Input: part model. Units: mm. Frame: model coordinates. Face numbers are marked on the shaded views. A direction names the side the tool comes from. Coordinates: 2 decimals unless noted, no trailing zeros. Order: outer loops, then holes, each group sorted by start corner. A loop starts at its lowest first (then second) coordinate and runs counter-clockwise, first axis right, second up. Notation, with made-up numbers: (77, 84.25) -> (99, 84.25) arc R33 ccw to (99, 113.25) -> close; hole circle Ø2 at (-28.75, 30). An arc over 180 degrees is marked (long way). Use one line per item in the form item = value. Start each with the question number.
1) Draft query along Z for the marked faces 5, 6, 7 and 8. Return one class per face: pulls with the +Z half, pulls with the -Z half, needs draft (parallel to the pull), parting line crosses it, or undercut.
2) Access query for the marked faces 1, 2, 3 and 4. Directions: +Z, -Z, +X, -X, +Y, -Y. A direction counts if a zero-diameter tool reaches every point of the face in a straight line with its end or side. Return the directions, or none.
3) Section query C-C on z = 25.5. Output: boundary loops of the cut face in (x, y) (3 decimals), then the cut area to 3 significant figures.
4) Pin query (flat end, axial travel): pin 1 (12 mm diameter, centred on y = 9.5, z = 20, fed in from -X); pin 2 (12 mm diameter, centred on y = 15, z = -1.5, fed in from -X); pin 3 (4 mm diameter, centred on x = 7.5, z = 14.47, fed in from -Y); pin 4 (4 mm diameter, centred on y = -6.5, z = 3.5, fed in from +X). Return the tip coordinate at first contact, or that it passes through.
5) Section query A-A on y = 5. Output: boundary loops of the cut face in (x, z), then the cut area to 4 significant figures.
6) Section query B-B on z = 4. Output: boundary loops of the cut face in (x, y) (3 decimals).
7) Ray query, line 1 along X through (y, z) = (15.5, -9); line 2 along Y through (x, z) = (-6.5, 26.5) (3 decimals); line 3 along X through (y, z) = (-4, -3.5). Return the intervals inside material, ascending.
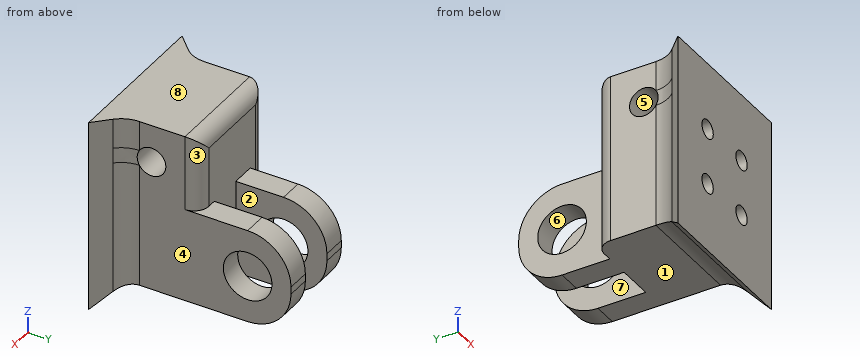
from build123d import *

# Parameters (mm, degrees)
SKETCH1_W                       = 28.58
SKETCH1_H                       = 50
BOSS_EXTRUDE1_DEPTH             = 12.5
SKETCH2_W                       = 9.53
SKETCH2_H                       = 24.225
SKETCH2_W_2                     = 6.35
CUT_EXTRUDE1_DEPTH              = 39.134028111
FILLET1_R                       = 11.53
SKETCH3_R                       = 6.477
CUT_EXTRUDE2_DEPTH              = 40.975822693
BOSS_EXTRUDE2_DEPTH             = 28.58
SKETCH5_W                       = 28.58
SKETCH5_H                       = 25.775
BOSS_EXTRUDE3_DEPTH             = 20
CUT_EXTRUDE3_DEPTH              = 50.98066026
CUT_EXTRUDE3_DEPTH_BACK         = 50.98066026
SKETCH6_R                       = 3.81
BOSS_EXTRUDE4_REACH             = 55.425
BOSS_EXTRUDE4_DIRECTION_2_REACH = 55.425
F_5_0MM_DOWEL_HOLE1_D           = 5
F_5_0MM_DOWEL_HOLE1_DEPTH       = 10
F_5_0MM_DOWEL_HOLE1_TIP         = 1.502151548
FILLET2_R                       = 8
FILLET4_R                       = 4


with BuildPart() as part:
    # Sketch1 → Boss-Extrude1 (new, symmetric)
    with BuildSketch(Plane.XY):
        Rectangle(SKETCH1_W, SKETCH1_H)
    extrude(amount=BOSS_EXTRUDE1_DEPTH, both=True)

    # Sketch2 → Cut-Extrude1 (cut, through all)
    with BuildSketch(Plane(origin=(0, 0, 12.5), x_dir=(-1, 0, 0), z_dir=(0, 0, 1))):
        with Locations((-3.175, -12.8875)):
            Rectangle(SKETCH2_W, SKETCH2_H)
        with Locations((11.115, -12.8875)):
            Rectangle(SKETCH2_W_2, SKETCH2_H)
    extrude(amount=-CUT_EXTRUDE1_DEPTH, mode=Mode.SUBTRACT)

    # Fillet1
    fillet1_edges = [part.edges().sort_by_distance(p)[0] for p in [
        (-4.765, 25, -12.5),
        (-4.765, 25, 12.5),
        (11.115, 25, -12.5),
        (11.115, 25, 12.5),
    ]]
    fillet(fillet1_edges, radius=FILLET1_R)

    # Sketch3 → Cut-Extrude2 (cut, through all)
    with BuildSketch(Plane(origin=(14.29, 0, 0), x_dir=(0, 0, -1), z_dir=(1, 0, 0))):
        with Locations(Location((0, 13.47, 0), (0, 0, 270))):
            Circle(SKETCH3_R)
    extrude(amount=-CUT_EXTRUDE2_DEPTH, mode=Mode.SUBTRACT)

    # Sketch4 → Boss-Extrude2 (add)
    with BuildSketch(Plane(origin=(14.29, 0, 0), x_dir=(0, 0, -1), z_dir=(1, 0, 0))):
        Polygon((18.85, -25), (12.5, -18.65), (12.5, -25), align=None)
    extrude(amount=-BOSS_EXTRUDE2_DEPTH)

    # Sketch5 → Boss-Extrude3 (add)
    with BuildSketch(Plane.XY.offset(12.5)):
        with Locations((0, -12.1125)):
            Rectangle(SKETCH5_W, SKETCH5_H)
    extrude(amount=BOSS_EXTRUDE3_DEPTH)

    # Sketch6 → Cut-Extrude3 (cut, two sides: drawn at the far end of the back side and taken through both)
    with BuildSketch(Plane(origin=(14.29, 0, 0), x_dir=(0, 0, -1), z_dir=(1, 0, 0)).offset(-CUT_EXTRUDE3_DEPTH_BACK)):
        with Locations((-22.5, -12.1125)):
            Circle(SKETCH6_R)
    extrude(amount=CUT_EXTRUDE3_DEPTH + CUT_EXTRUDE3_DEPTH_BACK, mode=Mode.SUBTRACT)

    # Boss-Extrude4: up to this face of the body (flat: up to its plane)
    boss_extrude4_end = Plane(part.part.faces().sort_by_distance((0, -12.1125, 32.5))[0])
    # Sketch7 → Boss-Extrude4 (add, up to the picked face)
    with BuildSketch(Plane(origin=(0, 0, -12.5), x_dir=(-1, 0, 0), z_dir=(0, 0, -1)), mode=Mode.PRIVATE) as boss_extrude4_sk1:
        Polygon((-14.29, -25), (-20.64, -25), (-14.29, -18.65), align=None)
    boss_extrude4_tool1 = split(extrude(boss_extrude4_sk1.sketch, amount=-BOSS_EXTRUDE4_REACH, mode=Mode.PRIVATE), bisect_by=boss_extrude4_end, keep=Keep.BOTH, mode=Mode.PRIVATE)
    boss_extrude4 = boss_extrude4_tool1.solids().sort_by(Axis((16.406667, -22.883333, -12.5), (0, 0, 1)))[0]
    add(boss_extrude4)

    # Boss-Extrude4 direction 2: up to this face of the body (flat: up to its plane)
    boss_extrude4_direction_2_end = Plane(part.part.faces().sort_by_distance((0, -21.825, -15.675))[0])
    # Sketch7 → Boss-Extrude4 direction 2 (add, up to the picked face)
    with BuildSketch(Plane(origin=(0, 0, -12.5), x_dir=(-1, 0, 0), z_dir=(0, 0, -1)), mode=Mode.PRIVATE) as boss_extrude4_direction_2_sk1:
        Polygon((-14.29, -25), (-20.64, -25), (-14.29, -18.65), align=None)
    boss_extrude4_direction_2_tool1 = split(extrude(boss_extrude4_direction_2_sk1.sketch, amount=BOSS_EXTRUDE4_DIRECTION_2_REACH, mode=Mode.PRIVATE), bisect_by=boss_extrude4_direction_2_end, keep=Keep.BOTH, mode=Mode.PRIVATE)
    boss_extrude4_direction_2 = boss_extrude4_direction_2_tool1.solids().sort_by(Axis((16.406667, -22.883333, -12.5), (0, 0, -1)))[0]
    add(boss_extrude4_direction_2)

    # Mirror2: Boss-Extrude4, Boss-Extrude4 direction 2 across plane
    add(boss_extrude4.mirror(Plane(origin=(0, 0, 0), x_dir=(0, 0, 1), z_dir=(1, 0, 0))))
    add(boss_extrude4_direction_2.mirror(Plane(origin=(0, 0, 0), x_dir=(0, 0, 1), z_dir=(1, 0, 0))))

    # Ø5.0mm Dowel Hole1
    with Locations(Plane(origin=(0, -25, 0), x_dir=(-1, 0, 0), z_dir=(0, -1, 0))):
        with Locations((-7.5, 0.534345417), (7.5, 0.534345417), (7.5, -14.465654583), (-7.5, -14.465654583)):
            Hole(F_5_0MM_DOWEL_HOLE1_D / 2, depth=F_5_0MM_DOWEL_HOLE1_DEPTH)
            with Locations((0, 0, -(F_5_0MM_DOWEL_HOLE1_DEPTH + F_5_0MM_DOWEL_HOLE1_TIP / 2))):  # 118° drill point
                Cone(0, F_5_0MM_DOWEL_HOLE1_D / 2, F_5_0MM_DOWEL_HOLE1_TIP, mode=Mode.SUBTRACT)

    # Fillet2
    fillet2_edges = [part.edges().sort_by_distance(p)[0] for p in [
        (14.29, -18.65, 10),
        (-14.29, -18.65, 10),
        (0, -18.65, -12.5),
    ]]
    fillet(fillet2_edges, radius=FILLET2_R)

    # Fillet4
    fillet4_edges = [part.edges().sort_by_distance(p)[0] for p in [
        (-14.29, 0.775, 10),
        (14.29, 0.775, 22.5),
        (0, 0.775, 32.5),
    ]]
    fillet(fillet4_edges, radius=FILLET4_R)


solid = part.part
Answers below:
q1.face_5 = undercut
q1.face_6 = undercut
q1.face_7 = needs draft
q1.face_8 = pulls with the +Z half
q2.face_1 = -Z, +X, -X, +Y
q2.face_2 = +Z, -Z, +Y
q2.face_3 = +Z, +X, +Y
q2.face_4 = +Z, -Z, +X, +Y
q3.outline = (-20.64, -25) -> (20.64, -25) -> (16.633, -20.993) arc R8 cw to (14.29, -15.336) -> (14.29, -14.461) -> (-14.29, -14.461) -> (-14.29, -15.336) arc R8 cw to (-16.633, -20.993) -> close; (-14.29, -9.764) -> (14.29, -9.764) -> (14.29, -3.225) arc R4 ccw to (10.29, 0.775) -> (-10.29, 0.775) arc R4 ccw to (-14.29, -3.225) -> close
q3.area = 639 mm^2
q4.pin_1 = through
q4.pin_2 = -7.94
q4.pin_3 = -14.7
q4.pin_4 = 14.29
q5.outline = (-7.94, -12.5) -> (-1.59, -12.5) -> (-1.59, 12.5) -> (-7.94, 12.5) -> close; (7.94, -12.5) -> (14.29, -12.5) -> (14.29, 12.5) -> (7.94, 12.5) -> close
q5.area = 317.5 mm^2
q6.outline = (-20.64, -25) -> (20.64, -25) -> (16.633, -20.993) arc R8 cw to (14.29, -15.336) -> (14.29, 8.376) -> (7.94, 8.376) -> (7.94, 0.775) -> (-1.59, 0.775) -> (-1.59, 8.376) -> (-7.94, 8.376) -> (-7.94, 0.775) -> (-10.29, 0.775) arc R4 ccw to (-14.29, -3.225) -> (-14.29, -15.336) arc R8 cw to (-16.633, -20.993) -> close; (-7.94, 18.564) -> (-1.59, 18.564) -> (-1.59, 24.595) -> (-7.94, 24.595) -> close; (7.94, 18.564) -> (14.29, 18.564) -> (14.29, 24.595) -> (7.94, 24.595) -> close
q7.line_1 = -7.94 to -1.59, 7.94 to 14.29
q7.line_2 = -25 to 0.775
q7.line_3 = -14.29 to 14.29
